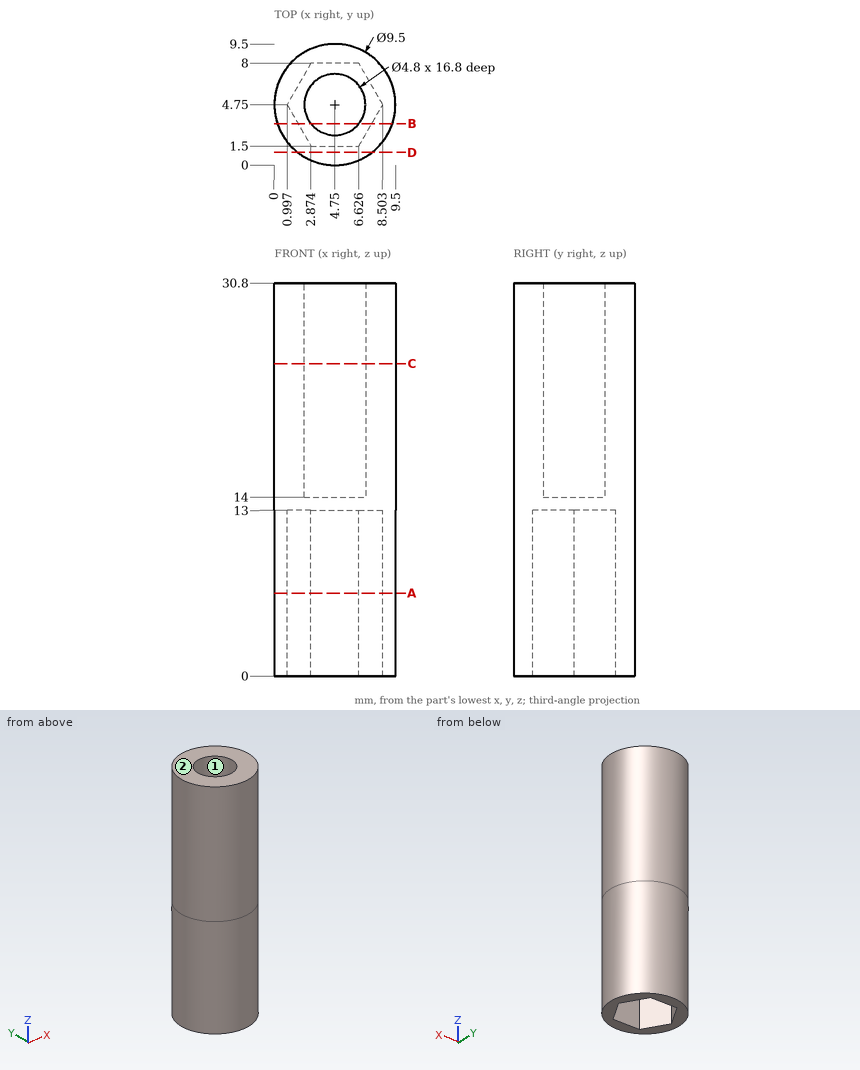
Design review of the part shown in the three views and the two pictorial views. Dimensions are in mm from the part's minimum x, y and z. Give positions to 0.01 mm unless a question says otherwise; leave off trailing zeros. Loops run counter-clockwise (first coordinate to the right, second up) from the corner with the lowest first, then second, coordinate; pieces in that order, holes last. Notation, with made-up numbers: (10.25, 48.5) - (38.25, 48.5) arc R18 ccw to (38.25, 63.5) - close; hole circle Ø3 at (-21.75, 31). An arc over 180 degrees is marked (long way). Answer as a JSON object with one key per item and string values.
Q1. To check wall thickness, follow line 1 along Y through (x, z) = (4.75, 22.25); line 2 along Z through (x, y) = (4.25, 5.5). State the ranges of each line that lie inside material, in increasing order.
Worked out:
{"line 1": "y = 0 to 2.35, 7.15 to 9.5", "line 2": "z = 13 to 14"}
Q2. Add section D-D on y = 1. State the section outline as (x, z) points (1 decimal).
Worked out:
{"outline": "(1.8, 0) - (7.7, 0) - (7.7, 30.8) - (1.8, 30.8) - close"}
Q3. Insertion check: pin 1 (5 mm diameter, centred on x = 1, z = 24, fed in from +Y); pin 2 (1.4 mm diameter, centred on x = 6, y = 5.5, fed in from +Z); pin 3 (3.5 mm diameter, centred on x = 4.5, y = 4, fed in from -Z); pin 4 (3 mm diameter, centred on x = 4.5, z = 7, fed in from +Y). Each pin has a flat end and moves straight along its axis. Give the tip position at first contact, or say it passes through.
Worked out:
{"pin 1": "stops at y = 9.33", "pin 2": "stops at z = 14", "pin 3": "stops at z = 13", "pin 4": "stops at y = 9.5"}
Q4. Add section A-A on z = 6.5. State the section outline as (x, y) points.
Worked out:
{"outline": "circle Ø9.5 at (4.75, 4.75); hole (1, 4.75) - (2.87, 1.5) - (6.63, 1.5) - (8.5, 4.75) - (6.63, 8) - (2.87, 8) - close"}
Q5. Mouldability with a two-part tool opening along X and no side actions: class the marked faces 1 and 2 as +X half, -X half, draft (parallel to the pull), parting line (faces both ways), or undercut.
Worked out:
{"face 1": "undercut", "face 2": "draft"}
Q6. Add section B-B on y = 3.25. State the section outline as (x, z) points.
Worked out:
{"outline": "(0.24, 0) - (1.86, 0) - (1.86, 13) - (7.64, 13) - (7.64, 0) - (9.26, 0) - (9.26, 30.8) - (6.62, 30.8) - (6.62, 14) - (2.88, 14) - (2.88, 30.8) - (0.24, 30.8) - close"}
Q7. Add section C-C on z = 24.5. State the section outline as (x, y) points, plus the area to 3 significant figures.
Worked out:
{"outline": "circle Ø9.5 at (4.75, 4.75); hole circle Ø4.8 at (4.75, 4.75)", "area": "52.8 mm^2"}
